Autodesk Inventor part; units mm, degrees
ref_plane "YZ Plane" through (0, 0, 0) normal (1, 0, 0) x (0, 1, 0)
ref_plane "XZ Plane" through (0, 0, 0) normal (0, 1, 0) x (-1, 0, 0)
ref_plane "XY Plane" through (0, 0, 0) normal (0, 0, 1) x (1, 0, 0)
sketch "Sketch1" plane through (0, 0, 0) normal (0, 0, 1) x (1, 0, 0)
  line L0 (0, 19.6828) -> (0, -18.3172)
  line L1 (-0.377, 15.178) -> (-10, 15.178)
  line L2 (-10, 15.178) -> (-5, 10.178)
  line L3 (-5, 10.178) -> (-5, -14.822)
  line L4 (-5, -14.822) -> (0, -14.822)
  line L5 (0, -14.822) -> (0, 15.178)
  line L6 (-0.377, 15.178) -> (0, 15.178)
  dimension "d2" = 20
  dimension "d3" = 45
  dimension "d4" = 30
  dimension "d6" = 10
revolve "Revolution1" add sketch "Sketch1" angle 360 about axis through (0, 19.6828, 0) along (0, -1, 0)
chamfer "Chamfer1" distance 1 angle 45 1 edges at (5, -14.822, 0)
sketch "Sketch2" plane through (0, 0, 0) normal (1, 0, 0) x (0, 1, 0)
  line L0 (-13.822, 5) -> (10.178, 5)
  line L1 (-13.822, -5) -> (10.178, -5)
  line L2 (-13.822, 5) -> (-13.322, 4)
  line L3 (-13.322, 4) -> (-12.822, 5)
  line L4 (-13.822, 5) -> (-12.822, 5)
  line L5 (-12.622, 0) -> (13.978, 0)
  dimension "d10" = 1
  dimension "d12" = 1
revolve "Revolution2" cut sketch "Sketch2" angle 360 about axis through (0, -10, 0) along (0, 1, 0)
pattern_linear "Rectangular Pattern1" count 15 spacing 1 along (0, 1, 0) of "Revolution2"
sketch "Sketch3" plane through (0, 15.178, 0) normal (0, 1, 0) x (1, 0, 0)
  circle A0 centre (0, 0) radius 10
  line L0 (1.7321, -3) -> (-1.7321, -3)
  line L1 (-1.7321, -3) -> (-3.4641, 0)
  line L2 (-3.4641, 0) -> (-1.7321, 3)
  line L3 (-1.7321, 3) -> (1.7321, 3)
  line L4 (1.7321, 3) -> (3.4641, 0)
  line L5 (3.4641, 0) -> (1.7321, -3)
  dimension "d17" = 6
extrude "Extrusion1" cut sketch "Sketch3" against normal blind 5 contours L0 L1 L2 L3 L4 L5
properties part number "M10x30 Allen Frezato"
Read the model definition and answer for the solid it produces. Units are mm, in the model's axes. Coordinates: 2 decimals unless noted, no trailing zeros. Loops run counter-clockwise (first coordinate to the right, second up) from the corner with the lowest first, then second, coordinate; pieces in that order, holes last. Notation, with made-up numbers: (-25.75, 77) - (-16.75, 77) arc R16 ccw to (-16.75, 97) - close; hole circle Ø6 at (41, 68.25). An arc over 180 degrees is marked (long way). Answer in a Markdown table with one row per item.
Q1. Straight lines are drawn through the part: line 1 along Z through (x, y) = (3.5, 10.5); line 2 along X through (y, z) = (7.75, 0); line 3 along Y through (x, z) = (1, -1). For each, find the intervals that lie inside material, in ascending order. Write a range as [from, to].
Here are the results:
| item | result |
|---|---|
| line 1 | z = [-4.01, 4.01] |
| line 2 | x = [-5, 5] |
| line 3 | y = [-14.82, 10.18] |
Q2. Find section A-A on y = 13.5. Write down the section's boundary in (x, z).
Here are the results:
| item | result |
|---|---|
| outline | circle Ø16.64 at (0, 0); hole (-3.46, 0) - (-1.73, -3) - (1.73, -3) - (3.46, 0) - (1.73, 3) - (-1.73, 3) - close |
Q3. The mould has two halves that part along Z. Classify faces 1 (the conical face through (1.152, 10.491, -5.186)), 2 (the flat face through (0, 13, 3)): pulls with the +Z half, pulls with the -Z half, needs draft (parallel to the pull), parting line crosses it, or undercut.
Here are the results:
| item | result |
|---|---|
| face 1 | parting line crosses it |
| face 2 | undercut |
Q4. Given P1, Ø1.7, axis at x = -0.5, y = 13, coming from the +Z side; P2, Ø8, axis at x = 6, y = 11.5, coming from the +Z side; P3, Ø1.8, axis at x = 0, z = -1, coming from the +Y side, each flat-ended and moving along its own axis, determine where each tip first touches the part or whether it passes through.
Here are the results:
| item | result |
|---|---|
| P1 | stops at z = 8.66 |
| P2 | stops at z = 8.97 |
| P3 | stops at y = 10.18 |
Q5. Find section B-B on x = 4.5. Count the separate pieces of the cut face and the enclosed holes in it, plus the area to 3 significant figures.
Here are the results:
| item | result |
|---|---|
| separate pieces | 16 |
| enclosed holes | 0 |
| area | 121 mm^2 |
